```python
from build123d import *

# Parameters (mm, degrees)
F1_DEPTH     = 5.08
F2_DEPTH     = 8.89
F3_T1_DEPTH  = 11.0681121842
F3_T3_DEPTH  = 11.0681121842
F3_T5_DEPTH  = 11.0681121842
F3_T7_DEPTH  = 11.0681121842
F3_T9_DEPTH  = 11.0681121842
F3_T11_DEPTH = 11.0681121842
F3_T13_DEPTH = 11.0681121842
F3_T15_DEPTH = 11.0681121842
F3_T17_DEPTH = 11.0681121842
F3_T19_DEPTH = 11.0681121842
F3_T21_DEPTH = 11.0681121842
F3_T23_DEPTH = 11.0681121842
F3_T25_DEPTH = 11.0681121842
F3_T27_DEPTH = 11.0681121842
F3_T29_DEPTH = 11.0681121842
F3_T31_DEPTH = 11.0681121842
F4_R         = 5.08
F5_DEPTH     = 3.81
F6_R         = 3.80999
F7_R         = 1.27
F8_DEPTH     = 1.27
F9_R         = 1.26999


# Not quite as in the source:
# - a fillet or chamfer that OpenCascade refuses, or shapes differently, is made with other operations: its cross-section is extruded or revolved along the edge and cut away or added
# - a fillet or chamfer is up to 0.001 mm smaller than in the source, because OpenCascade refuses the exact size
# - a feature names something its author has since deleted; it is built from what else it names


with BuildPart() as f1:
    # F0 (on Top) → F1 (new body)
    with BuildSketch(Plane.XY):
        with BuildLine():
            Line((8.255, 0), (9.525, 0))
            ThreePointArc((9.525, 0), (9.3419797958, 1.8582353172), (8.7999525472, 3.6450596933))
            Line((8.7999525472, 3.6450596933), (7.6266255409, 3.1590517342))
            ThreePointArc((7.6266255409, 3.1590517342), (6.8637816496, 4.5862322736), (5.8371664787, 5.8371664787))
            Line((5.8371664787, 5.8371664787), (6.7351920908, 6.7351920908))
            ThreePointArc((6.7351920908, 6.7351920908), (5.2918064695, 7.9197480572), (3.6450596933, 8.7999525472))
            Line((3.6450596933, 8.7999525472), (3.1590517342, 7.6266255409))
            ThreePointArc((3.1590517342, 7.6266255409), (1.6104706082, 8.0963824897), (0, 8.255))
            Line((0, 8.255), (0, 9.525))
            ThreePointArc((0, 9.525), (-1.8582353172, 9.3419797958), (-3.6450596933, 8.7999525472))
            Line((-3.6450596933, 8.7999525472), (-3.1590517342, 7.6266255409))
            ThreePointArc((-3.1590517342, 7.6266255409), (-4.5862322736, 6.8637816496), (-5.8371664787, 5.8371664787))
            Line((-5.8371664787, 5.8371664787), (-6.7351920908, 6.7351920908))
            ThreePointArc((-6.7351920908, 6.7351920908), (-7.9197480572, 5.2918064695), (-8.7999525472, 3.6450596933))
            Line((-8.7999525472, 3.6450596933), (-7.6266255409, 3.1590517342))
            ThreePointArc((-7.6266255409, 3.1590517342), (-8.0963824897, 1.6104706082), (-8.255, 0))
            Line((-8.255, 0), (-9.525, 0))
            ThreePointArc((-9.525, 0), (-9.3419797958, -1.8582353172), (-8.7999525472, -3.6450596933))
            Line((-8.7999525472, -3.6450596933), (-7.6266255409, -3.1590517342))
            ThreePointArc((-7.6266255409, -3.1590517342), (-6.8637816496, -4.5862322736), (-5.8371664787, -5.8371664787))
            Line((-5.8371664787, -5.8371664787), (-6.7351920908, -6.7351920908))
            ThreePointArc((-6.7351920908, -6.7351920908), (-5.2918064695, -7.9197480572), (-3.6450596933, -8.7999525472))
            Line((-3.6450596933, -8.7999525472), (-3.1590517342, -7.6266255409))
            ThreePointArc((-3.1590517342, -7.6266255409), (-1.6104706082, -8.0963824897), (0, -8.255))
            Line((0, -8.255), (0, -9.525))
            ThreePointArc((0, -9.525), (1.8582353172, -9.3419797958), (3.6450596933, -8.7999525472))
            Line((3.6450596933, -8.7999525472), (3.1590517342, -7.6266255409))
            ThreePointArc((3.1590517342, -7.6266255409), (4.5862322736, -6.8637816496), (5.8371664787, -5.8371664787))
            Line((5.8371664787, -5.8371664787), (6.7351920908, -6.7351920908))
            ThreePointArc((6.7351920908, -6.7351920908), (7.9197480572, -5.2918064695), (8.7999525472, -3.6450596933))
            Line((8.7999525472, -3.6450596933), (7.6266255409, -3.1590517342))
            ThreePointArc((7.6266255409, -3.1590517342), (8.0963824897, -1.6104706082), (8.255, 0))
        make_face()
        with BuildLine():
            ThreePointArc((-8.7999525472, -3.6450596933), (-7.9197480572, -5.2918064695), (-6.7351920908, -6.7351920908))
            Line((-6.7351920908, -6.7351920908), (-5.8371664787, -5.8371664787))
            ThreePointArc((-5.8371664787, -5.8371664787), (-6.8637816496, -4.5862322736), (-7.6266255409, -3.1590517342))
            Line((-7.6266255409, -3.1590517342), (-8.7999525472, -3.6450596933))
        make_face()
    extrude(amount=F1_DEPTH)

    # F0 (on Top) → F2 (join)
    with BuildSketch(Plane.XY):
        with BuildLine():
            Line((3.1590517342, 7.6266255409), (3.6450596933, 8.7999525472))
            ThreePointArc((3.6450596933, 8.7999525472), (1.8582353172, 9.3419797958), (0, 9.525))
            Line((0, 9.525), (0, 8.255))
            ThreePointArc((0, 8.255), (1.6104706082, 8.0963824897), (3.1590517342, 7.6266255409))
        make_face()
        with BuildLine():
            Line((7.6266255409, 3.1590517342), (8.7999525472, 3.6450596933))
            ThreePointArc((8.7999525472, 3.6450596933), (7.9197480572, 5.2918064695), (6.7351920908, 6.7351920908))
            Line((6.7351920908, 6.7351920908), (5.8371664787, 5.8371664787))
            ThreePointArc((5.8371664787, 5.8371664787), (6.8637816496, 4.5862322736), (7.6266255409, 3.1590517342))
        make_face()
        with BuildLine():
            ThreePointArc((3.6450596933, -8.7999525472), (5.2918064695, -7.9197480572), (6.7351920908, -6.7351920908))
            Line((6.7351920908, -6.7351920908), (5.8371664787, -5.8371664787))
            ThreePointArc((5.8371664787, -5.8371664787), (4.5862322736, -6.8637816496), (3.1590517342, -7.6266255409))
            Line((3.1590517342, -7.6266255409), (3.6450596933, -8.7999525472))
        make_face()
        with BuildLine():
            ThreePointArc((8.7999525472, -3.6450596933), (9.3419797958, -1.8582353172), (9.525, 0))
            Line((9.525, 0), (8.255, 0))
            ThreePointArc((8.255, 0), (8.0963824897, -1.6104706082), (7.6266255409, -3.1590517342))
            Line((7.6266255409, -3.1590517342), (8.7999525472, -3.6450596933))
        make_face()
        with BuildLine():
            ThreePointArc((-3.6450596933, -8.7999525472), (-1.8582353172, -9.3419797958), (0, -9.525))
            Line((0, -9.525), (0, -8.255))
            ThreePointArc((0, -8.255), (-1.6104706082, -8.0963824897), (-3.1590517342, -7.6266255409))
            Line((-3.1590517342, -7.6266255409), (-3.6450596933, -8.7999525472))
        make_face()
        with BuildLine():
            ThreePointArc((-8.7999525472, -3.6450596933), (-7.9197480572, -5.2918064695), (-6.7351920908, -6.7351920908))
            Line((-6.7351920908, -6.7351920908), (-5.8371664787, -5.8371664787))
            ThreePointArc((-5.8371664787, -5.8371664787), (-6.8637816496, -4.5862322736), (-7.6266255409, -3.1590517342))
            Line((-7.6266255409, -3.1590517342), (-8.7999525472, -3.6450596933))
        make_face()
        with BuildLine():
            Line((-7.6266255409, 3.1590517342), (-8.7999525472, 3.6450596933))
            ThreePointArc((-8.7999525472, 3.6450596933), (-9.3419797958, 1.8582353172), (-9.525, 0))
            Line((-9.525, 0), (-8.255, 0))
            ThreePointArc((-8.255, 0), (-8.0963824897, 1.6104706082), (-7.6266255409, 3.1590517342))
        make_face()
        with BuildLine():
            Line((-3.1590517342, 7.6266255409), (-3.6450596933, 8.7999525472))
            ThreePointArc((-3.6450596933, 8.7999525472), (-5.2918064695, 7.9197480572), (-6.7351920908, 6.7351920908))
            Line((-6.7351920908, 6.7351920908), (-5.8371664787, 5.8371664787))
            ThreePointArc((-5.8371664787, 5.8371664787), (-4.5862322736, 6.8637816496), (-3.1590517342, 7.6266255409))
        make_face()
    extrude(amount=F2_DEPTH)

    # F3: chamfer of 1.905 on 16 edges, made by hand

    # F3_s2 → F3_t1 (cut)
    with BuildSketch(Plane(origin=(1.2842641335, 3.1004878888, 0), x_dir=(0, 0, 1), z_dir=(0.3826834324, 0.9238795325, 0))):
        Polygon((8.89, -1.905), (6.985, 0), (8.89, 0), align=None)
    extrude(amount=F3_T1_DEPTH, mode=Mode.SUBTRACT)

    # F3_s4 → F3_t3 (cut)
    with BuildSketch(Plane.XZ.offset(-14.4240560921)):
        Polygon((0, 6.985), (1.905, 8.89), (0, 8.89), align=None)
    extrude(amount=F3_T3_DEPTH, mode=Mode.SUBTRACT)

    # F3_s6 → F3_t5 (cut)
    with BuildSketch(Plane(origin=(3.1004878888, 1.2842641335, 0), x_dir=(0, 0, 1), z_dir=(0.9238795325, 0.3826834324, 0))):
        Polygon((8.89, -1.905), (6.985, 0), (8.89, 0), align=None)
    extrude(amount=F3_T5_DEPTH, mode=Mode.SUBTRACT)

    # F3_s8 → F3_t7 (cut)
    with BuildSketch(Plane(origin=(10.1993478749, 10.1993478749, 0), x_dir=(0, 0, 1), z_dir=(-0.7071067812, -0.7071067812, 0))):
        Polygon((6.985, 0), (8.89, -1.905), (8.89, 0), align=None)
    extrude(amount=F3_T7_DEPTH, mode=Mode.SUBTRACT)

    # F3_s10 → F3_t9 (cut)
    with BuildSketch(Plane(origin=(1.2842641335, -3.1004878888, 0), x_dir=(0, 0, 1), z_dir=(0.3826834324, -0.9238795325, 0))):
        Polygon((8.89, -1.905), (6.985, 0), (8.89, 0), align=None)
    extrude(amount=F3_T9_DEPTH, mode=Mode.SUBTRACT)

    # F3_s12 → F3_t11 (cut)
    with BuildSketch(Plane(origin=(10.1993478749, -10.1993478749, 0), x_dir=(0, 0, 1), z_dir=(-0.7071067812, 0.7071067812, 0))):
        Polygon((6.985, 0), (8.89, -1.905), (8.89, 0), align=None)
    extrude(amount=F3_T11_DEPTH, mode=Mode.SUBTRACT)

    # F3_s14 → F3_t13 (cut)
    with BuildSketch(Plane(origin=(3.1004878888, -1.2842641335, 0), x_dir=(0, 0, 1), z_dir=(0.9238795325, -0.3826834324, 0))):
        Polygon((8.89, -1.905), (6.985, 0), (8.89, 0), align=None)
    extrude(amount=F3_T13_DEPTH, mode=Mode.SUBTRACT)

    # F3_s16 → F3_t15 (cut)
    with BuildSketch(Plane.YZ.offset(3.3559439079)):
        Polygon((0, 6.985), (-1.905, 8.89), (0, 8.89), align=None)
    extrude(amount=F3_T15_DEPTH, mode=Mode.SUBTRACT)

    # F3_s18 → F3_t17 (cut)
    with BuildSketch(Plane.XZ.offset(3.3559439079)):
        Polygon((0, 6.985), (-1.905, 8.89), (0, 8.89), align=None)
    extrude(amount=F3_T17_DEPTH, mode=Mode.SUBTRACT)

    # F3_s20 → F3_t19 (cut)
    with BuildSketch(Plane(origin=(-1.2842641335, -3.1004878888, 0), x_dir=(0, 0, 1), z_dir=(-0.3826834324, -0.9238795325, 0))):
        Polygon((8.89, -1.905), (6.985, 0), (8.89, 0), align=None)
    extrude(amount=F3_T19_DEPTH, mode=Mode.SUBTRACT)

    # F3_s22 → F3_t21 (cut)
    with BuildSketch(Plane(origin=(-10.1993478749, -10.1993478749, 0), x_dir=(0, 0, 1), z_dir=(0.7071067812, 0.7071067812, 0))):
        Polygon((6.985, 0), (8.89, -1.905), (8.89, 0), align=None)
    extrude(amount=F3_T21_DEPTH, mode=Mode.SUBTRACT)

    # F3_s24 → F3_t23 (cut)
    with BuildSketch(Plane(origin=(-3.1004878888, -1.2842641335, 0), x_dir=(0, 0, 1), z_dir=(-0.9238795325, -0.3826834324, 0))):
        Polygon((8.89, -1.905), (6.985, 0), (8.89, 0), align=None)
    extrude(amount=F3_T23_DEPTH, mode=Mode.SUBTRACT)

    # F3_s26 → F3_t25 (cut)
    with BuildSketch(Plane.YZ.offset(-14.4240560921)):
        Polygon((0, 6.985), (1.905, 8.89), (0, 8.89), align=None)
    extrude(amount=F3_T25_DEPTH, mode=Mode.SUBTRACT)

    # F3_s28 → F3_t27 (cut)
    with BuildSketch(Plane(origin=(-3.1004878888, 1.2842641335, 0), x_dir=(0, 0, 1), z_dir=(-0.9238795325, 0.3826834324, 0))):
        Polygon((8.89, -1.905), (6.985, 0), (8.89, 0), align=None)
    extrude(amount=F3_T27_DEPTH, mode=Mode.SUBTRACT)

    # F3_s30 → F3_t29 (cut)
    with BuildSketch(Plane(origin=(-10.1993478749, 10.1993478749, 0), x_dir=(0, 0, 1), z_dir=(0.7071067812, -0.7071067812, 0))):
        Polygon((6.985, 0), (8.89, -1.905), (8.89, 0), align=None)
    extrude(amount=F3_T29_DEPTH, mode=Mode.SUBTRACT)

    # F3_s32 → F3_t31 (cut)
    with BuildSketch(Plane(origin=(-1.2842641335, 3.1004878888, 0), x_dir=(0, 0, 1), z_dir=(-0.3826834324, 0.9238795325, 0))):
        Polygon((8.89, -1.905), (6.985, 0), (8.89, 0), align=None)
    extrude(amount=F3_T31_DEPTH, mode=Mode.SUBTRACT)

    # F4 (on face) → F5 (join)
    with BuildSketch(Plane.XY.offset(5.08)):
        Circle(F4_R)
    extrude(amount=F5_DEPTH)

    # F6 (radius 3.81 in the source; OpenCascade refuses exactly that, so slightly less here)
    f6_edges = [f1.edges().sort_by_distance(p)[0] for p in [
        (-5.08, 0, 8.89),
    ]]
    fillet(f6_edges, radius=F6_R)

    # F7 (on face) → F8 (join)
    with BuildSketch(Plane.XY.offset(8.89)):
        Circle(F7_R)
    extrude(amount=F8_DEPTH)

    # F9 (radius 1.27 in the source; OpenCascade refuses exactly that, so slightly less here)
    f9_edges = [f1.edges().sort_by_distance(p)[0] for p in [
        (-1.27, 0, 10.16),
    ]]
    fillet(f9_edges, radius=F9_R)


solid = f1.part
```
Design review of the part built by this model. Coordinates are the model's own, in mm. A direction names the side the tool comes from. Give positions to 0.01 mm unless a question says otherwise; leave off trailing zeros. Order: outer loops, then holes, each group sorted by start corner. A loop starts at its lowest first (then second) coordinate and runs counter-clockwise, first axis right, second up. Notation, with made-up numbers: (-37.75, -29.75) -> (-27.75, -29.75) arc R8 cw to (-27.75, -18.75) -> close; hole circle Ø8 at (-1, -10). An arc over 180 degrees is marked (long way). Write each question's results on one line, items separated by ' | '. Start each with the question number.
Q1. Wall thickness on L1, parallel to Z at x = -4, y = 6.25; L2, parallel to X at y = -4.75, z = 4: over which ranges is each line inside the solid? List them lowest first. Write a range as from..to.
Q2. For pin 1 (1.3 mm diameter, centred on x = 0.5, y = 0.5, fed in from +Z); pin 2 (3 mm diameter, centred on x = -7, z = 8, fed in from -Y); pin 3 (0.6 mm diameter, centred on x = 9, z = 6, fed in from +Y); pin 4 (1 mm diameter, centred on y = 8.5, z = 6.5, fed in from -X), all flat-tipped, find the tip position at first contact; note any pin that passes through.
Q3. Machinability: for faces 1 (the flat face through (3.4, -8.21, 6.02)), 2 (the flat face through (9, 0, 6)), 3 (the cylindrical face through (4.61, -6.85, 6.42)), which of the approach directions +Z, -Z, +X, -X, +Y, -Y give a long, thin tool a straight path to every point of the face, cutting with its end or side? Answer none if there is none.
Q4. Add section B-B on x = -7.25. Give the boundary of the cut face in (y, z).
Q5. Add section A-A on z = 4.25. Give the boundary of the cut face in (x, y) (3 decimals).
Found:
1) L1: z = 0..5.08 | L2: x = -8.26..8.26
2) pin 1: stops at z = 10.16 | pin 2: stops at y = -6.74 | pin 3: stops at y = 3.88 | pin 4: stops at x = -5.17
3) face 1: +Z, -Y | face 2: +Z, +X | face 3: +Z
4) outline: (-6.18, 0) -> (6.18, 0) -> (6.18, 5.08) -> (-3.95, 5.08) -> (-3.95, 7.86) -> (-4.84, 8.69) -> (-6.18, 7.74) -> close
5) outline: circle Ø19.05 at (0, 0)
